from build123d import *

# Parameters (mm, degrees)
SKETCH5_W               = 160
SKETCH5_H               = 100
BOSS_EXTRUDE2_DEPTH     = 20
SKETCH6_W               = 51
SKETCH6_H               = 15
CUT_EXTRUDE1_DEPTH      = 1
CUT_EXTRUDE1_DEPTH_BACK = 21
SKETCH7_R               = 6
BOSS_EXTRUDE3_DEPTH     = 50
SKETCH8_R               = 5
CUT_EXTRUDE2_DEPTH      = 15.5
CUT_EXTRUDE2_DEPTH_BACK = 86.5
BOSS_EXTRUDE4_DEPTH     = 4
BOSS_EXTRUDE5_DEPTH     = 5


with BuildPart() as part:
    # Sketch5 → Boss-Extrude2 (new body)
    with BuildSketch(Plane.XY):
        with Locations((-1155.707372839, 36.928751241)):
            Rectangle(SKETCH5_W, SKETCH5_H)
        Polygon((-1065.42313354, 5.690501508), (-1075.707372839, -13.071248759), (-1075.707372839, 86.928751241), (-1066.90354904, 72.432300318), align=None)
        with BuildLine():
            Line((-1235.707372839, 86.928751241), (-1235.707372839, -13.071248759))
            ThreePointArc((-1235.707372839, -13.071248759), (-1256.717577983, 36.928751241), (-1235.707372839, 86.928751241))
        make_face()
    extrude(amount=BOSS_EXTRUDE2_DEPTH)

    # Sketch6 → Cut-Extrude1 (cut, two sides)
    with BuildSketch(Plane.XY.offset(20)) as cut_extrude1_sk:
        with Locations((-1195.595351444, -6.071248759)):
            Rectangle(SKETCH6_W, SKETCH6_H)
        with Locations((-1195.595351444, 79.928751241)):
            Rectangle(SKETCH6_W, SKETCH6_H)
    extrude(amount=CUT_EXTRUDE1_DEPTH, mode=Mode.SUBTRACT)
    extrude(cut_extrude1_sk.sketch, amount=-CUT_EXTRUDE1_DEPTH_BACK, mode=Mode.SUBTRACT)

    # Sketch7 → Boss-Extrude3 (add)
    with BuildSketch(Plane(origin=(0, 0, 0), x_dir=(-1, 0, 0), z_dir=(0, 0, -1))):
        with Locations((1079.344915198, 64.512007402)):
            Circle(SKETCH7_R)
        with Locations((1079.344915198, 9.345495081)):
            Circle(SKETCH7_R)
        with Locations((1232.069830479, 9.345495081)):
            Circle(SKETCH7_R)
        with Locations((1232.069830479, 64.512007402)):
            Circle(SKETCH7_R)
    extrude(amount=BOSS_EXTRUDE3_DEPTH)

    # Sketch8 → Cut-Extrude2 (cut, two sides)
    with BuildSketch(Plane.XZ.offset(-1.428751241)) as cut_extrude2_sk:
        with Locations((-1195.095351444, 10)):
            Circle(SKETCH8_R)
    extrude(amount=CUT_EXTRUDE2_DEPTH, mode=Mode.SUBTRACT)
    extrude(cut_extrude2_sk.sketch, amount=-CUT_EXTRUDE2_DEPTH_BACK, mode=Mode.SUBTRACT)

    # Sketch9 → Boss-Extrude4 (add)
    with BuildSketch(Plane(origin=(0, 0, 0), x_dir=(-1, 0, 0), z_dir=(0, 0, -1))):
        with BuildLine():
            Line((1165.095351444, 6.428751241), (1226.095351444, 6.428751241))
            Line((1226.095351444, 6.428751241), (1226.095351444, -8.071248759))
            Line((1226.095351444, -8.071248759), (1233.621735581, -8.071248759))
            ThreePointArc((1233.621735581, -8.071248759), (1251.717577983, 36.928751241), (1233.621735581, 81.928751241))
            Line((1233.621735581, 81.928751241), (1226.095351444, 81.928751241))
            Line((1226.095351444, 81.928751241), (1226.095351444, 67.428751241))
            Line((1226.095351444, 67.428751241), (1165.095351444, 67.428751241))
            Line((1165.095351444, 67.428751241), (1165.095351444, 81.928751241))
            Line((1165.095351444, 81.928751241), (1078.520666135, 81.928751241))
            Line((1078.520666135, 81.928751241), (1071.872609564, 70.982004916))
            Line((1071.872609564, 70.982004916), (1070.451613888, 6.919039109))
            Line((1070.451613888, 6.919039109), (1078.668528909, -8.071248759))
            Line((1078.668528909, -8.071248759), (1165.095351444, -8.071248759))
            Line((1165.095351444, -8.071248759), (1165.095351444, 6.428751241))
        make_face()
    extrude(amount=BOSS_EXTRUDE4_DEPTH)

    # Sketch10 → Boss-Extrude5 (add)
    with BuildSketch(Plane(origin=(0, 0, 0), x_dir=(-1, 0, 0), z_dir=(0, 0, -1))):
        with BuildLine():
            Line((1170.095351444, 1.428751241), (1221.095351444, 1.428751241))
            Line((1221.095351444, 1.428751241), (1221.095351444, -13.071248759))
            Line((1221.095351444, -13.071248759), (1235.707372839, -13.071248759))
            ThreePointArc((1235.707372839, -13.071248759), (1256.717577983, 36.928751241), (1235.707372839, 86.928751241))
            Line((1235.707372839, 86.928751241), (1221.095351444, 86.928751241))
            Line((1221.095351444, 86.928751241), (1221.095351444, 72.428751241))
            Line((1221.095351444, 72.428751241), (1170.095351444, 72.428751241))
            Line((1170.095351444, 72.428751241), (1170.095351444, 86.928751241))
            Line((1170.095351444, 86.928751241), (1075.707372839, 86.928751241))
            Line((1075.707372839, 86.928751241), (1066.90354904, 72.432300318))
            Line((1066.90354904, 72.432300318), (1065.42313354, 5.690501508))
            Line((1065.42313354, 5.690501508), (1075.707372839, -13.071248759))
            Line((1075.707372839, -13.071248759), (1170.095351444, -13.071248759))
            Line((1170.095351444, -13.071248759), (1170.095351444, 1.428751241))
        make_face()
    extrude(amount=-BOSS_EXTRUDE5_DEPTH)


solid = part.part
Can you work these out from the model? Positions are in its coordinate system, mm. A direction names the side the tool comes from. Give positions to 0.01 mm unless a question says otherwise; leave off trailing zeros. Order: outer loops, then holes, each group sorted by start corner. A loop starts at its lowest first (then second) coordinate and runs counter-clockwise, first axis right, second up. Notation, with made-up numbers: M 75,34 L 96,34 A6 cw 96,44 Z; hole C -32.75,89.5 d2. An arc over 180 degrees is marked long. Use a Markdown table: item, result. Add a question column.
Item 1: Suppose I cut it at D-D (y = -5). List the corners of the cut face in (x, z) for me, then the cut area to 3 significant figures.
Item 2: Suppose I cut it at B-B (x = -1204). List the corners of the cut face in (y, z) for me.
Item 3: Suppose I cut it at A-A (z = 10). List the corners of the cut face in (x, y) for me, then the cut area to 3 significant figures.
Item 4: For faces 5 (the flat face through (-1230, -8.071, -2)), 6 (the flat face through (-1074.5, -0.47, -1.97)), 7 (the flat face through (-1122, 81.929, -2)), 8 (the flat face through (-1165.095, 75, -2)), 9 (the flat face through (-1195, 6.429, -2)), which set-ups out of +Z, -Z, +X, -X, +Y, -Y let a thin tool reach every point of the face, with its end or its side?
Item 5: Suppose I cut it at C-C (y = 56.5). List the corners of the cut face in (x, z) for me.
Item 6: Will these pins go through, and if not, where does the flat tip stop? pin 1 (11.5 mm diameter, centred on y = -9.5, z = 8.5, fed in from -X); pin 2 (2 mm diameter, centred on x = -1137, z = -2, fed in from +Y); pin 3 (11.5 mm diameter, centred on y = 80.5, z = 13.5, fed in from +X); pin 4 (6 mm diameter, centred on x = -1195.1, z = 10, fed in from +Y).
Item 7: We'd pull the mould along Y, two halves only. Please class faces 1 (the cylindrical face through (-1073.35, 9.61, -26.68)), 2 (the flat face through (-1079, 9, -50)), 3 (the flat face through (-1229, -13.071, 10)), 4 (the flat face through (-1230, 81.929, -2)): +Y half, -Y half, draft (parallel to the pull), parting line (faces both ways), or undercut.
Item 8: If I drill on L1, parallel to Z at x = -1164, y = 47; L2, parallel to X at y = 65.5, z = -28; L3, parallel to X at y = 19, z = 10, over which ranges is the centre line in solid material (lowest first)? Write a range as [from, to].
Answer sheet:
| question | item | result |
|---|---|---|
| 1 | outline | M -1242.77,0 L -1236.39,0 L -1236.39,-4 L -1226.1,-4 L -1226.1,0 L -1221.1,0 L -1221.1,20 L -1242.77,20 Z; M -1170.1,0 L -1165.1,0 L -1165.1,-4 L -1076.99,-4 L -1076.99,0 L -1071.28,0 L -1071.28,20 L -1170.1,20 Z |
| 1 | area | 2,800 mm² |
| 2 | outline | M 1.43,0 L 6.43,0 L 6.43,-4 L 67.43,-4 L 67.43,0 L 72.43,0 L 72.43,20 L 1.43,20 Z |
| 3 | outline | M -1235.71,-13.07 L -1221.1,-13.07 L -1221.1,1.43 L -1200.1,1.43 L -1200.1,72.43 L -1221.1,72.43 L -1221.1,86.93 L -1235.71,86.93 A70 ccw Z; M -1190.1,1.43 L -1170.1,1.43 L -1170.1,-13.07 L -1075.71,-13.07 L -1065.42,5.69 L -1066.9,72.43 L -1075.71,86.93 L -1170.1,86.93 L -1170.1,72.43 L -1190.1,72.43 Z |
| 3 | area | 16,100 mm² |
| 4 | face 5 | -Z, +X, -X, -Y |
| 4 | face 6 | -Z, +X, -Y |
| 4 | face 7 | -Z, +X, -X, +Y |
| 4 | face 8 | -Z, +Y |
| 4 | face 9 | -Z, -Y |
| 5 | outline | M -1253.93,0 L -1248.7,0 L -1248.7,-4 L -1071.55,-4 L -1071.55,0 L -1066.55,0 L -1066.55,20 L -1253.93,20 Z; hole C -1195.1,10 d10 |
| 6 | pin 1 | stops at x = -1243.68 |
| 6 | pin 2 | stops at y = 81.93 |
| 6 | pin 3 | stops at x = -1068.31 |
| 6 | pin 4 | passes through |
| 7 | face 1 | undercut |
| 7 | face 2 | draft |
| 7 | face 3 | -Y half |
| 7 | face 4 | +Y half |
| 8 | L1 | z = [-4, 20] |
| 8 | L2 | x = [-1237.99, -1226.15], [-1085.26, -1073.43] |
| 8 | L3 | x = [-1254.38, -1200.1], [-1190.1, -1065.72] |
